Print and shaded views of the part. All mm, measured from the part's lowest x, y and z. Coordinates: 2 decimals unless noted, no trailing zeros. Order: outer loops, then holes, each group sorted by start corner. A loop starts at its lowest first (then second) coordinate and runs counter-clockwise, first axis right, second up. Notation, with made-up numbers: M 16,-31.5 L 37,-31.5 A17 ccw 37,-19.5 Z; hole C -9.5,-19.5 d7. An arc over 180 degrees is marked long. One line per item, written item: value.
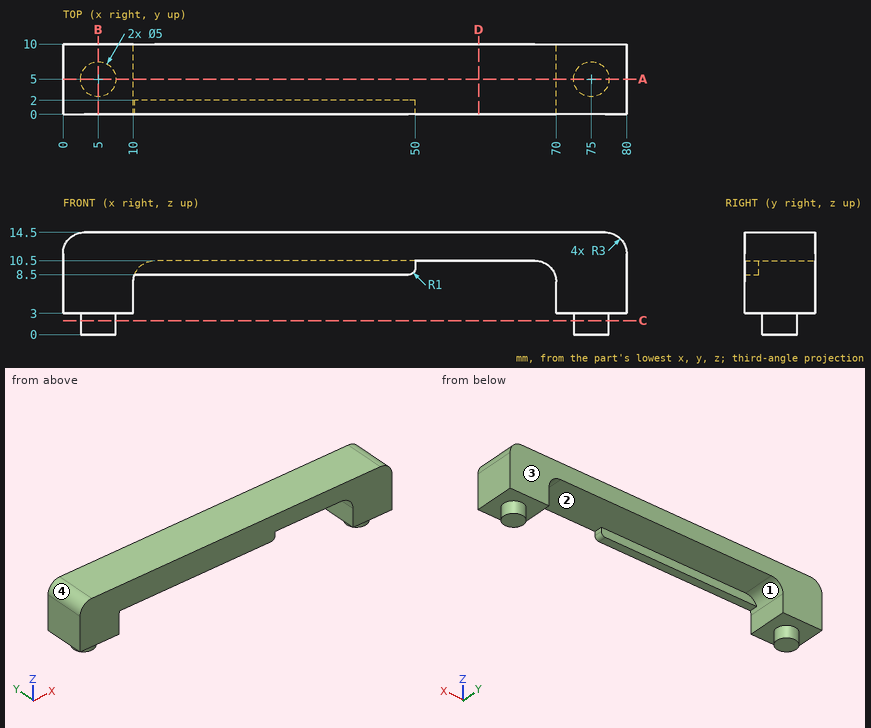
Q1. Slice it at A-A (y = 5). List the corners of the cut face in (x, z).
Recorded:
outline: M 0,3 L 2.5,3 L 2.5,0 L 7.5,0 L 7.5,3 L 10,3 L 10,7.5 A3 cw 13,10.5 L 67,10.5 A3 cw 70,7.5 L 70,3 L 72.5,3 L 72.5,0 L 77.5,0 L 77.5,3 L 80,3 L 80,11.5 A3 ccw 77,14.5 L 3,14.5 A3 ccw 0,11.5 Z
Q2. Slice it at C-C (z = 2). List the corners of the cut face in (x, y), plus the area to 3 significant figures.
Recorded:
outline: C 5,5 d5; C 75,5 d5
area: 39.3 mm^2
Q3. Slice it at D-D (x = 59). List the corners of the cut face in (y, z), plus the area to 3 significant figures.
Recorded:
outline: M 0,10.5 L 10,10.5 L 10,14.5 L 0,14.5 Z
area: 40.0 mm^2
Q4. Drill centre lines: line 1 along X through (y, z) = (1, 7.75); line 2 along Z through (x, y) = (48, 8.25); line 3 along Z through (x, y) = (28, 1.5). Where is each one in solid material? Low to high.
Recorded:
line 1: x = 0 to 10.01, 69.99 to 80
line 2: z = 10.5 to 14.5
line 3: z = 8.5 to 14.5
Q5. Pin check, flat tips, straight feed: pin 1 Ø5 at (x, y) = (30.5, 8.5) entering from -Z; pin 2 Ø1.6 at (x, y) = (21.5, 1.5) entering from -Z; pin 3 Ø3 at (x, z) = (42.5, 7.5) entering from +Y. Stop position of each tip, or through.
Recorded:
pin 1: stops at z = 10.5
pin 2: stops at z = 8.5
pin 3: stops at y = 2
Q6. Slice it at B-B (x = 5). List the corners of the cut face in (y, z), plus the area to 3 significant figures.
Recorded:
outline: M 0,3 L 2.5,3 L 2.5,0 L 7.5,0 L 7.5,3 L 10,3 L 10,14.5 L 0,14.5 Z
area: 130 mm^2
Q7. Mould opens along X. For the marked faces 1, 2, 3 and 4 say: released by +X, released by -X, zero draft, split by the parting line, or undercut.
Recorded:
face 1: undercut
face 2: undercut
face 3: zero draft
face 4: released by -X
